from build123d import *

# Parameters (mm, degrees)
BOSS_EXTRUDE4_DEPTH   = 7.62
BODY_MOVE_COPY4_ANGLE = 180
BOSS_EXTRUDE5_START   = -25.4
SKETCH2_R             = 9.5
BOSS_EXTRUDE5_DEPTH   = 146.02
LPATTERN1_COUNT       = 3
LPATTERN1_PITCH       = 146.02
BODY_MOVE_COPY5_ANGLE = 120
BODY_MOVE_COPY6_ANGLE = 120
BOSS_EXTRUDE6_START   = 27.92
SKETCH4_R             = 9.5
BOSS_EXTRUDE6_DEPTH   = 27.92


with BuildPart() as part:
    # Sketch1 → Boss-Extrude4 (new body)
    with BuildSketch(Plane(origin=(0, 0, 0), x_dir=(1, 0, 0), z_dir=(0, 1, 0))):
        with BuildLine():
            Line((-5.499261314, 15.875), (-10.998522628, 6.35))
            ThreePointArc((-10.998522628, 6.35), (0, -12.7), (10.998522628, 6.35))
            Line((10.998522628, 6.35), (5.499261314, 15.875))
            ThreePointArc((5.499261314, 15.875), (0, 19.05), (-5.499261314, 15.875))
        make_face()
    extrude(amount=BOSS_EXTRUDE4_DEPTH)


with BuildPart() as body_2:
    # Body-Move_Copy3: copy of part
    add(part.part.moved(Location((0, 60.96, 0))))


with BuildPart() as body_2_1:
    # Body-Move_Copy4: moved
    add(body_2.part.rotate(Axis((0, 0, 0), (0, 1, 0)), BODY_MOVE_COPY4_ANGLE))


with BuildPart() as part_1:
    add(part.part)

    add(body_2_1.part)  # Boss-Extrude5 merges body 2
    # Sketch2 → Boss-Extrude5 (add)
    with BuildSketch(Plane(origin=(0, 0, 0), x_dir=(1, 0, 0), z_dir=(0, 1, 0)).offset(BOSS_EXTRUDE5_START)):
        with Locations(Location((0, 0, 0), (0, 0, 270))):
            Circle(SKETCH2_R)
    extrude(amount=BOSS_EXTRUDE5_DEPTH)


with BuildPart() as lpattern1_1:
    # LPattern1: pattern copy
    add(part_1.part.moved(Location(Vector(0, 1, 0) * (1 * LPATTERN1_PITCH))))


with BuildPart() as lpattern1_2:
    # LPattern1: pattern copy
    add(part_1.part.moved(Location(Vector(0, 1, 0) * (2 * LPATTERN1_PITCH))))


with BuildPart() as lpattern1_1_1:
    # Body-Move_Copy5: moved
    add(lpattern1_1.part.rotate(Axis((0, 0, 0), (0, 1, 0)), BODY_MOVE_COPY5_ANGLE))


with BuildPart() as lpattern1_2_1:
    # Body-Move_Copy6: moved
    add(lpattern1_2.part.rotate(Axis((0, 0, 0), (0, -1, 0)), BODY_MOVE_COPY6_ANGLE))


with BuildPart() as part_2:
    add(part_1.part)

    # Sketch4 → Boss-Extrude6 (add)
    with BuildSketch(Plane.XZ.offset(25.4).offset(BOSS_EXTRUDE6_START)):
        with Locations(Location((0, 0, 0), (0, 0, 90))):
            Circle(SKETCH4_R)
    extrude(amount=-BOSS_EXTRUDE6_DEPTH)


with BuildPart() as lpattern1_2_2:
    add(lpattern1_2_1.part)

    # Combine1: union LPattern1_1, part
    add(lpattern1_1_1.part)
    add(part_2.part)


solid = lpattern1_2_2.part
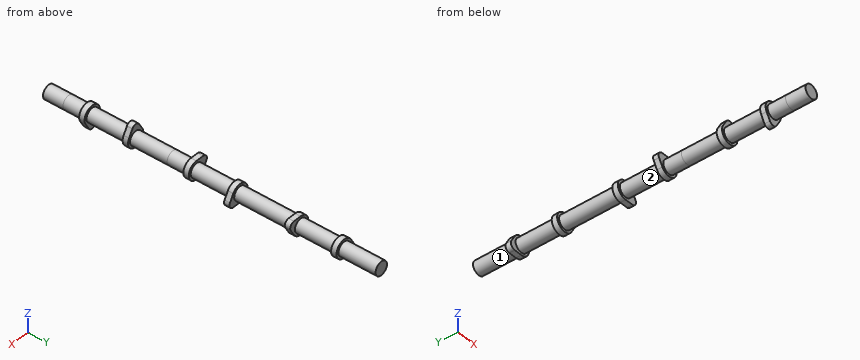
Verification items for the finished model (mm, model axes). Face numbers are marked on the shaded views. Round coordinates to 2 decimals unless told otherwise and drop trailing zeros. Loops run counter-clockwise (first coordinate to the right, second up) from the corner with the lowest first, then second, coordinate; pieces in that order, holes last. Notation, with made-up numbers: (33.5, -24.75) - (92.5, -24.75) arc R33 cw to (92.5, 4.25) - close; hole circle Ø10 at (-2, -7.75). An arc over 180 degrees is marked (long way). Answer in a Markdown table with one row per item. Add a question column.
Q1. Gauge pin test, flat ends, axial feed: pin 1 (3 mm diameter, centred on y = 211, z = 0, fed in from +X); pin 2 (8 mm diameter, centred on y = 62, z = 1.5, fed in from -X); pin 3 (3 mm diameter, centred on x = -8, z = -13.5, fed in from +Y); pin 4 (20.5 mm diameter, centred on x = 9, z = 3.5, fed in from +Y). Record the tip position at first contact, or that the pin passes through.
Q2. Section check A-A on y = 102. Enter the section's corners in (x, z), plus the area to 3 significant figures.
Q3. Material ranges on line 1 (Y direction, x = -4.5, z = 9); line 2 (Y direction, x = -11.5, z = 10.5); line 3 (X direction, y = 389, z = 0), recorded low to high.
Q4. Release check for a two-part mould opening along Y. For the marked faces 1 and 2 record: pulls with the +Y half, pulls with the -Y half, needs draft (parallel to the pull), parting line crosses it, or undercut.
Found:
| question | item | result |
|---|---|---|
| 1 | pin 1 | stops at x = 15.53 |
| 1 | pin 2 | stops at x = -12.7 |
| 1 | pin 3 | stops at y = 360.62 |
| 1 | pin 4 | stops at y = 412.66 |
| 2 | outline | circle Ø19 at (0, 0) |
| 2 | area | 284 mm² |
| 3 | line 1 | y = 0 to 7.62, 60.96 to 68.58, 146.02 to 153.64, 206.98 to 214.6, 292.04 to 299.66, 353 to 360.62 |
| 3 | line 2 | y = 146.02 to 153.64 |
| 3 | line 3 | x = -9.5 to 9.5 |
| 4 | face 1 | needs draft |
| 4 | face 2 | undercut |
